Check sheet for the modelled part. Datum: model origin and axes. Units: mm. A direction names the side the tool comes from. Give positions to 0.01 mm unless a question says otherwise; leave off trailing zeros. Order: outer loops, then holes, each group sorted by start corner. A loop starts at its lowest first (then second) coordinate and runs counter-clockwise, first axis right, second up.
from build123d import *

# Parameters (mm, degrees)
SURFACE_SKETCH_W       = 22.5
SURFACE_SKETCH_H       = 30
BODY_DEPTH             = 4.5
SKETCH_19_W            = 22.5
SKETCH_19_H            = 24
EXTRUDE_4_DEPTH        = 3
FILLET_6_R             = 1.5
MAGNET_CUTOUT_SKETCH_W = 2.2
MAGNET_CUTOUT_SKETCH_H = 6.2
MAGNET_CUTOUT_DEPTH    = 2.6
BORDER_DEPTH           = 0.5
CHAMPFER_DEPTH         = 22.5
FILLET_7_R             = 1.5
FILLET_8_R             = 0.5
CUT_EXTRUDE_1_DEPTH    = 23.5


with BuildPart() as part:
    # surface_sketch → body (new body)
    with BuildSketch(Plane(origin=(0, 0, 0), x_dir=(1, 0, 0), z_dir=(0, 1, 0))):
        with Locations((-1.15, 0)):
            Rectangle(SURFACE_SKETCH_W, SURFACE_SKETCH_H)
    extrude(amount=-BODY_DEPTH)

    # Эскиз19 → Бобышка-Вытянуть4 (add)
    with BuildSketch(Plane(origin=(0, -4.5, 0), x_dir=(1, 0, 0), z_dir=(0, 1, 0))):
        with Locations((-1.15, -27)):
            Rectangle(SKETCH_19_W, SKETCH_19_H)
    extrude(amount=EXTRUDE_4_DEPTH)

    # Скругление6
    fillet_6_edges = [part.edges().sort_by_distance(p)[0] for p in [
        (-12.4, -3, 39),
        (10.1, -3, 39),
        (10.1, -2.25, -15),
        (-12.4, -2.25, -15),
    ]]
    fillet(fillet_6_edges, radius=FILLET_6_R)

    # magnet_cutout_sketch → magnet_cutout (cut)
    with BuildSketch(Plane.XZ.offset(4.5)):
        with Locations((9, 7.1)):
            Rectangle(MAGNET_CUTOUT_SKETCH_W, MAGNET_CUTOUT_SKETCH_H)
    magnet_cutout = extrude(amount=-MAGNET_CUTOUT_DEPTH, mode=Mode.SUBTRACT)

    # magnet_cutout_mirror: magnet_cutout across plane
    add(magnet_cutout.mirror(Plane(origin=(-1.15, 0, 0), x_dir=(0, 0, 1), z_dir=(1, 0, 0))), mode=Mode.SUBTRACT)

    # border_sketch → border (add)
    with BuildSketch(Plane(origin=(0, 0, 0), x_dir=(1, 0, 0), z_dir=(0, 1, 0))):
        with BuildLine():
            Line((-12.4, -15), (-12.4, 13.5))
            ThreePointArc((-12.4, 13.5), (-11.960660172, 14.560660172), (-10.9, 15))
            Line((-10.9, 15), (8.6, 15))
            ThreePointArc((8.6, 15), (9.660660172, 14.560660172), (10.1, 13.5))
            Line((10.1, 13.5), (10.1, -15))
            Line((10.1, -15), (9.1, -15))
            Line((9.1, -15), (9.1, 13.5))
            ThreePointArc((9.1, 13.5), (8.953553391, 13.853553391), (8.6, 14))
            Line((8.6, 14), (-10.9, 14))
            ThreePointArc((-10.9, 14), (-11.253553391, 13.853553391), (-11.4, 13.5))
            Line((-11.4, 13.5), (-11.4, -15))
            Line((-11.4, -15), (-12.4, -15))
        make_face()
    extrude(amount=BORDER_DEPTH)

    # Эскиз21 → champfer (add)
    with BuildSketch(Plane.ZY.offset(12.4)):
        Polygon((15, 0.5), (17, -1.5), (15, -1.5), (14, -1.5), (14, 0.5), align=None)
    extrude(amount=-CHAMPFER_DEPTH)

    # Скругление7
    fillet_7_edges = [part.edges().sort_by_distance(p)[0] for p in [
        (-12.4, -0.5, 16),
        (10.1, -0.5, 16),
    ]]
    fillet(fillet_7_edges, radius=FILLET_7_R)

    # Скругление8
    fillet_8_edges = [part.edges().sort_by_distance(p)[0] for p in [
        (9.1, 0.25, 14),
        (-11.4, 0.25, 14),
    ]]
    fillet(fillet_8_edges, radius=FILLET_8_R)

    # Эскиз22 → Вырез-Вытянуть1 (cut, through all)
    with BuildSketch(Plane.ZY.offset(12.4)):
        with BuildLine():
            Line((12.878679656, 0.5), (14.378679656, 0.5))
            ThreePointArc((14.378679656, 0.5), (14.952704805, 0.385819299), (15.439339828, 0.060660172))
            Line((15.439339828, 0.060660172), (17, -1.5))
            Line((17, -1.5), (17.923275361, -1.5))
            Line((17.923275361, -1.5), (15.181180077, 1.242095285))
            Line((15.181180077, 1.242095285), (12.878679656, 1.122407091))
            Line((12.878679656, 1.122407091), (12.878679656, 0.5))
        make_face()
    extrude(amount=-CUT_EXTRUDE_1_DEPTH, mode=Mode.SUBTRACT)


solid = part.part
1) Section check A-A, the plane y = -3.25. Record the cut outline in (x, z), then the cut area to 3 significant figures.
Recorded:
outline: (-12.4, -13.5) arc R1.5 ccw to (-10.9, -15) - (8.6, -15) arc R1.5 ccw to (10.1, -13.5) - (10.1, 4) - (7.9, 4) - (7.9, 10.2) - (10.1, 10.2) - (10.1, 37.5) arc R1.5 ccw to (8.6, 39) - (-10.9, 39) arc R1.5 ccw to (-12.4, 37.5) - (-12.4, 10.2) - (-10.2, 10.2) - (-10.2, 4) - (-12.4, 4) - close
area: 1,190 mm2
2) Set-up check for faces 4 (the face through (9, -1.9, 7)), 5 (the face through (-10.2, -3, 7)), 6 (the face through (-1, 0, 0)), 7 (the face through (9.67, -2.98, 38.55)), 8 (the face through (9.649, -0.294, 15.189)): record each of +Z, -Z, +X, -X, +Y, -Y from which the full face is reachable in a straight line by a thin tool's end or side.
Recorded:
face 4: +X, -Y
face 5: -X, -Y
face 6: +Y
face 7: +Z, +X, +Y, -Y
face 8: +Z, +X, +Y
3) Section check C-C, the plane x = -9.5. Record the cut outline in (y, z).
Recorded:
outline: (-4.5, -15) - (0.5, -15) - (0.5, -14) - (0, -14) - (0, 14) - (0.5, 14) - (0.5, 14.38) arc R1.5 ccw to (0.06, 15.44) - (-1.5, 17) - (-1.5, 39) - (-4.5, 39) - close
4) Depth check by flat-ended pin: pin 1 Ø1.8 at (x, z) = (9.5, 8.5) entering from -Y; pin 2 Ø10 at (x, z) = (7.5, 11) entering from +Y; pin 3 Ø11 at (x, z) = (2.5, 30) entering from +Y; pin 4 Ø0.8 at (y, z) = (-2.5, 8) entering from +X. Enter the tip coordinate at first touch or a pass-through.
Recorded:
pin 1: stops at y = -1.9
pin 2: stops at y = 0.5
pin 3: stops at y = -1.5
pin 4: stops at x = 7.9
5) Material ranges on L1, parallel to Z at x = 8, y = -3.6; L2, parallel to Y at x = -7, z = 25.5; L3, parallel to Y at x = -3, z = 3, recorded low to high.
Recorded:
L1: z = -15 to 4, 10.2 to 39
L2: y = -4.5 to -1.5
L3: y = -4.5 to 0
6) Section check B-B, the plane z = 2. Record the cut outline in (x, y), then the cut area to 3 significant figures.
Recorded:
outline: (-12.4, -4.5) - (10.1, -4.5) - (10.1, 0.5) - (9.1, 0.5) - (9.1, 0) - (-11.4, 0) - (-11.4, 0.5) - (-12.4, 0.5) - close
area: 102 mm2
7) Section check D-D, the plane z = 31. Record the cut outline in (x, y), then the cut area to 3 significant figures.
Recorded:
outline: (-12.4, -4.5) - (10.1, -4.5) - (10.1, -1.5) - (-12.4, -1.5) - close
area: 67.5 mm2
8) Draft check along Z on faces 1 (the face through (-1, -1.5, 27)), 2 (the face through (-11.97, -2.04, -14.55)), 3 (the face through (-11, -3, 10.2)). Enter one of: +Z half, -Z half, draft (parallel to the pull), parting line (faces both ways), or undercut.
Recorded:
face 1: draft
face 2: -Z half
face 3: undercut
